from build123d import *

# Parameters (mm, degrees)
RESSALTO_EXTRUS_O1_DEPTH = 3
ESBO_O3_W                = 10
ESBO_O3_H                = 3
ESBO_O3_W_2              = 3
ESBO_O3_H_2              = 10
ESBO_O3_W_3              = 3.017337907
CORTE_EXTRUS_O1_DEPTH    = 3
ESBO_O4_W                = 30
ESBO_O4_H                = 70
CORTE_EXTRUS_O2_DEPTH    = 3


with BuildPart() as part:
    # Esboço1 → Ressalto-extrusão1 (new body)
    with BuildSketch(Plane(origin=(0, 0, 0), x_dir=(1, 0, 0), z_dir=(0, 1, 0))):
        Polygon((-97.357643635, -26.698729811), (-97.357643635, 73.301270189), (102.642356365, 73.301270189), (102.642356365, -26.698729811), (77.642356365, -70), (-72.357643635, -70), align=None)
    extrude(amount=RESSALTO_EXTRUS_O1_DEPTH)

    # Esboço3 → Corte-extrusão1 (cut)
    with BuildSketch(Plane(origin=(0, 3, 0), x_dir=(1, 0, 0), z_dir=(0, 1, 0))):
        with Locations((-62.357643635, -63.5)):
            Rectangle(ESBO_O3_W, ESBO_O3_H)
        with Locations((67.642356365, -63.5)):
            Rectangle(ESBO_O3_W, ESBO_O3_H)
        with Locations((96.142356365, -11.698729811)):
            Rectangle(ESBO_O3_W_2, ESBO_O3_H_2)
        with Locations((96.133687412, 58.301270189)):
            Rectangle(ESBO_O3_W_3, ESBO_O3_H_2)
        with Locations((92.642356365, 66.801270189)):
            Rectangle(ESBO_O3_W, ESBO_O3_H)
        with Locations((-90.857643635, -11.698729811)):
            Rectangle(ESBO_O3_W_2, ESBO_O3_H_2)
        with Locations((-90.857643635, 58.301270189)):
            Rectangle(ESBO_O3_W_2, ESBO_O3_H_2)
        with Locations((-87.357643635, 66.801270189)):
            Rectangle(ESBO_O3_W, ESBO_O3_H)
    extrude(amount=-CORTE_EXTRUS_O1_DEPTH, mode=Mode.SUBTRACT)

    # Esboço4 → Corte-extrusão2 (cut)
    with BuildSketch(Plane(origin=(0, 3, 0), x_dir=(1, 0, 0), z_dir=(0, 1, 0))):
        with Locations((-67.357643635, 18.301270189)):
            Rectangle(ESBO_O4_W, ESBO_O4_H)
        with Locations((72.642356365, 18.301270189)):
            Rectangle(ESBO_O4_W, ESBO_O4_H)
    extrude(amount=-CORTE_EXTRUS_O2_DEPTH, mode=Mode.SUBTRACT)


solid = part.part
Check sheet for the modelled part. Datum: model origin and axes. Units: mm. Round coordinates to 2 decimals unless told otherwise and drop trailing zeros. Loops run counter-clockwise (first coordinate to the right, second up) from the corner with the lowest first, then second, coordinate; pieces in that order, holes last.
1. Scan lines: probe 1 along X at (y, z) = (1, 16.5); probe 2 along Z at (x, y) = (68.5, 1); probe 3 along X at (y, z) = (0.35, -67). Record each from-to range of solid material in increasing order.
2. Gauge pin test, flat ends, axial feed: pin 1 Ø1.5 at (y, z) = (2, 64) entering from +X; pin 2 Ø0.9 at (y, z) = (2, 63) entering from -X. Record the tip position at first contact, or that the pin passes through.
3. Sectioned sample at B-B on x = 65. Record the boundary of the cut face in (y, z), and give its area (3 significant figures).
4. Sectioned sample at C-C on z = -21.5. Record the boundary of the cut face in (x, y).
5. Sectioned sample at D-D on y = 0.7. Give the number of separate pieces and of enclosed holes in the cut face, and give its area (3 significant figures).
6. Sectioned sample at A-A on z = 13. Record the boundary of the cut face in (x, y).
Recorded:
1. probe 1: x = -97.36 to -92.36, -89.36 to -82.36, -52.36 to 57.64, 87.64 to 94.64, 97.64 to 102.64
1. probe 2: z = -73.3 to -53.3, 16.7 to 62, 65 to 70
1. probe 3: x = -97.36 to -92.36, -82.36 to 87.64, 97.64 to 102.64
2. pin 1: stops at x = 81.54
2. pin 2: stops at x = -76.66
3. outline: (0, -73.3) - (3, -73.3) - (3, -53.3) - (0, -53.3) - close; (0, 16.7) - (3, 16.7) - (3, 62) - (0, 62) - close; (0, 65) - (3, 65) - (3, 70) - (0, 70) - close
3. area: 211 mm2
4. outline: (-97.36, 0) - (-82.36, 0) - (-82.36, 3) - (-97.36, 3) - close; (-52.36, 0) - (57.64, 0) - (57.64, 3) - (-52.36, 3) - close; (87.64, 0) - (102.64, 0) - (102.64, 3) - (87.64, 3) - close
5. separate pieces: 1
5. enclosed holes: 10
5. area: 23,100 mm2
6. outline: (-97.36, 0) - (-92.36, 0) - (-92.36, 3) - (-97.36, 3) - close; (-89.36, 0) - (-82.36, 0) - (-82.36, 3) - (-89.36, 3) - close; (-52.36, 0) - (57.64, 0) - (57.64, 3) - (-52.36, 3) - close; (87.64, 0) - (94.64, 0) - (94.64, 3) - (87.64, 3) - close; (97.64, 0) - (102.64, 0) - (102.64, 3) - (97.64, 3) - close
